```python
from build123d import *

# Parameters (mm, degrees)
SKETCH_1_R          = 11.5
EXTRUDE_1_DEPTH     = 14
SKETCH_2_R          = 4
CUT_EXTRUDE_1_DEPTH = 24
SKETCH_3_R          = 10
SKETCH_3_R_2        = 5.5
CUT_EXTRUDE_2_DEPTH = 0.4
SKETCH_4_R          = 10
SKETCH_4_R_2        = 5.5
CUT_EXTRUDE_3_DEPTH = 0.4
CHAMFER_1_SIZE      = 0.2


with BuildPart() as part:
    # 草图1 → 凸台-拉伸1 (new body)
    with BuildSketch(Plane(origin=(0, 0, 0), x_dir=(1, 0, 0), z_dir=(0, 1, 0))):
        Circle(SKETCH_1_R)
    extrude(amount=EXTRUDE_1_DEPTH)

    # 草图2 → 切除-拉伸1 (cut)
    with BuildSketch(Plane(origin=(0, 14, 0), x_dir=(1, 0, 0), z_dir=(0, 1, 0))):
        Circle(SKETCH_2_R)
    extrude(amount=-CUT_EXTRUDE_1_DEPTH, mode=Mode.SUBTRACT)

    # 草图3 → 切除-拉伸2 (cut)
    with BuildSketch(Plane(origin=(0, 14, 0), x_dir=(1, 0, 0), z_dir=(0, 1, 0))):
        Circle(SKETCH_3_R)
        Circle(SKETCH_3_R_2, mode=Mode.SUBTRACT)
    extrude(amount=-CUT_EXTRUDE_2_DEPTH, mode=Mode.SUBTRACT)

    # 草图4 → 切除-拉伸3 (cut)
    with BuildSketch(Plane.XZ):
        Circle(SKETCH_4_R)
        Circle(SKETCH_4_R_2, mode=Mode.SUBTRACT)
    extrude(amount=-CUT_EXTRUDE_3_DEPTH, mode=Mode.SUBTRACT)

    # 倒角1
    chamfer_1_edges = [part.edges().sort_by_distance(p)[0] for p in [
        (-10, 14, 0),
        (-5.5, 14, 0),
        (-11.5, 0, 0),
        (-10, 0, 0),
        (-5.5, 0, 0),
        (-11.5, 14, 0),
        (-4, 0, 0),
        (-4, 14, 0),
    ]]
    chamfer(chamfer_1_edges, length=CHAMFER_1_SIZE)


solid = part.part
```
Input: part model. Units: mm. Frame: model coordinates. Coordinates: 2 decimals unless noted, no trailing zeros. Order: outer loops, then holes, each group sorted by start corner. A loop starts at its lowest first (then second) coordinate and runs counter-clockwise, first axis right, second up. Notation, with made-up numbers: (81.25, 10.25) - (103.25, 10.25) arc R24 ccw to (103.25, 35.25) - close; hole circle Ø2 at (83.25, 56). An arc over 180 degrees is marked (long way). Return JSON: item names as keys, results as strings.
Q1. First-contact query: pin 1 (8 mm diameter, centred on y = 4.5, z = 1.5, fed in from +X); pin 2 (6 mm diameter, centred on x = 7.5, y = 6, fed in from +Z); pin 3 (6 mm diameter, centred on y = 4.5, z = 5.5, fed in from -X) (3 decimals); pin 4 (4 mm diameter, centred on x = -8, y = 9.5, fed in from +Z). Flat tips, straight axial feed; report the tip coordinate or a pass-through.
The answers:
{"pin 1": "stops at x = 11.5", "pin 2": "stops at z = 10.58", "pin 3": "stops at x = -11.225", "pin 4": "stops at z = 9.81"}
Q2. Draft query along X for faces 1 (the flat face through (4, 0.4, -4)), 2 (the cylindrical face through (-1.5, 6.9, -11.4)), 3 (the flat face through (4, 13.6, 4)), 4 (the flat face through (-2, 0, -4)). Return one class per face: +X half, -X half, draft (parallel to the pull), parting line (faces both ways), or undercut.
The answers:
{"face 1": "undercut", "face 2": "parting line", "face 3": "undercut", "face 4": "draft"}
Q3. Ray query, probe 1 along X at (y, z) = (13.7, 0); probe 2 along Z at (x, y) = (0, 0.45). Return the intervals inside material, ascending.
The answers:
{"probe 1": "x = -11.5 to -10, -5.5 to -4, 4 to 5.5, 10 to 11.5", "probe 2": "z = -11.5 to -4, 4 to 11.5"}
Q4. Cut plane A-A (y = 11.5). Return loops of the section in (x, z), then the cut area to 3 significant figures.
The answers:
{"outline": "circle Ø23 at (0, 0); hole circle Ø8 at (0, 0)", "area": "365 mm2"}
